Read the model definition and answer for the solid it produces. Units are mm, in the model's axes. Give positions to 0.01 mm unless a question says otherwise; leave off trailing zeros. Write each loop counter-clockwise with the first axis right and the second up, starting at its lowest first coordinate (ties: lowest second). Pieces come first, ordered by that corner, then holes. Notation, with made-up numbers: (64.25, 77.5) - (104.25, 77.5) arc R18 ccw to (104.25, 91.5) - close; hole circle Ø8 at (4, -36). An arc over 180 degrees is marked (long way). Answer as a JSON object with one key per item and string values. Group by question number.
```python
from build123d import *

# Parameters (mm, degrees)
SKETCH_R           = 65.25
PAD_DEPTH          = 6
SKETCH001_R        = 5.5
POCKET_DEPTH       = 6.001
SKETCH002_R        = 2
POCKET001_DEPTH    = 375.305752
POLARPATTERN_COUNT = 3
CHAMFER_SIZE       = 1
FILLET_R           = 6
SKETCH003_R        = 63
POCKET002_DEPTH    = 3


with BuildPart() as part:
    # Sketch → Pad (new body)
    with BuildSketch(Plane.XY):
        Circle(SKETCH_R)
    extrude(amount=PAD_DEPTH)

    # Sketch001 → Pocket (cut, through all)
    with BuildSketch(Plane.XY):
        Circle(SKETCH001_R)
    extrude(amount=POCKET_DEPTH, mode=Mode.SUBTRACT)

    # Sketch002 → Pocket001 (cut, through all)
    with BuildSketch(Plane.XY):
        with Locations((0, 50)):
            Circle(SKETCH002_R)
        with BuildLine():
            ThreePointArc((-5, 59.791304), (-51.961524, 30), (-54.280788, -25.565525))
            Line((-10, 0), (-54.280788, -25.565525))
            ThreePointArc((-5, 8.660254), (-8.660254, 5), (-10, 0))
            Line((-5, 8.660254), (-5, 59.791304))
        make_face()
    pocket001 = extrude(amount=POCKET001_DEPTH, mode=Mode.SUBTRACT)

    # PolarPattern: Pocket001 ×3 about axis
    polarpattern_axis = Axis((0, 0, 0), (0, 0, 1))
    for i in range(1, POLARPATTERN_COUNT):
        add(pocket001.rotate(polarpattern_axis, i * 360 / POLARPATTERN_COUNT), mode=Mode.SUBTRACT)

    # Chamfer
    chamfer_edges = [part.edges().sort_by_distance(p)[0] for p in [
        (-65.25, 0, 6),
        (-65.25, 0, 0),
    ]]
    chamfer(chamfer_edges, length=CHAMFER_SIZE)

    # Fillet
    fillet_edges = [part.edges().sort_by_distance(p)[0] for p in [
        (-54.280788, -25.565525, 3),
        (-5, 59.791304, 3),
        (5, 59.791304, 3),
        (54.280788, -25.565525, 3),
        (49.280788, -34.225779, 3),
        (-49.280788, -34.225779, 3),
    ]]
    fillet(fillet_edges, radius=FILLET_R)

    # Sketch003 (on Face25 of Fillet) → Pocket002 (cut)
    with BuildSketch(Plane.XY.offset(6)):
        Circle(SKETCH003_R)
    extrude(amount=-POCKET002_DEPTH, mode=Mode.SUBTRACT)


solid = part.part
```
1) Find section B-B, the plane z = 4.1. Write down the section's boundary in (x, y).
2) Flat-ended cylindrical pins translate along their axes: pin 1 Ø2.5 at (y, z) = (32, 1.5) entering from -X; pin 2 Ø4.5 at (x, y) = (0, 50) entering from +Z; pin 3 Ø3.5 at (x, y) = (43.3, -25) entering from -Z; pin 4 Ø2.5 at (y, z) = (33.5, 1.5) entering from +X. Find the tip coordinate at first contact, or state that the pin passes through.
3) For a pull along X with two mould halves and no side action, classify faces 1 (the flat face through (43, -47, 6)), 2 (the cylindrical face through (46.22, -35.08, 1.52)), 3 (the cylindrical face through (-53.493, -22.487, 1.521)) as released by +X, released by -X, zero draft, split by the parting line, or undercut.
4) Find the intervals of material crossed by line 1 (Y direction, x = -12, z = 0.35); line 2 (X direction, y = 50, z = 2.1); line 3 (X direction, y = 20, z = 1.9), in increasing order. Write a range as [from, to].
5) Find section A-A, the plane x = 0. Write down the section's boundary in (y, z), and give its area (3 significant figures).
6) Find section C-C, the plane y = 50. Give the number of separate pieces and of enclosed holes in the cut face, and give its area (3 significant figures).
Values follow:
{
 "1": {"outline": "circle Ø130.5 at (0, 0); hole circle Ø126 at (0, 0)"},
 "2": {"pin 1": "stops at x = -57.55", "pin 2": "stops at z = 3", "pin 3": "passes through", "pin 4": "stops at x = 56.72"},
 "3": {"face 1": "zero draft", "face 2": "undercut", "face 3": "undercut"},
 "4": {"line 1": "y = [-63.48, -58.79], [-12.7, -1.15], [58.78, 63.48]", "line 2": "x = [-41.92, -33.17], [-5, -2], [2, 5], [33.17, 41.92]", "line 3": "x = [-62.11, -56.57], [-5, 5], [56.57, 62.11]"},
 "5": {"outline": "(-65.25, 1) - (-64.25, 0) - (-60, 0) - (-60, 3) - (-63, 3) - (-63, 6) - (-64.25, 6) - (-65.25, 5) - close; (-10, 0) - (-5.5, 0) - (-5.5, 3) - (-10, 3) - close; (5.5, 0) - (48, 0) - (48, 3) - (5.5, 3) - close; (52, 0) - (64.25, 0) - (65.25, 1) - (65.25, 5) - (64.25, 6) - (63, 6) - (63, 3) - (52, 3) - close", "area": "208 mm2"},
 "6": {"separate pieces": "4", "enclosed holes": "0", "area": "89.0 mm2"}
}
